```python
from build123d import *

# Parameters (mm, degrees)
M10_CLEARANCE_HOLE2_D                     = 11
M10_CLEARANCE_HOLE2_DEPTH                 = 55.695266595
M10_CLEARANCE_HOLE2_CSINK_D               = 11.05
M10_CLEARANCE_HOLE2_CSINK_ANGLE           = 90
M10_CLEARANCE_HOLE2_TIP                   = 3.304733405
M10_CLEARANCE_HOLE2_ON_FACE_2_D           = 11
M10_CLEARANCE_HOLE2_ON_FACE_2_DEPTH       = 55.695266595
M10_CLEARANCE_HOLE2_ON_FACE_2_CSINK_D     = 11.05
M10_CLEARANCE_HOLE2_ON_FACE_2_CSINK_ANGLE = 90
M10_CLEARANCE_HOLE2_ON_FACE_2_TIP         = 3.304733405
CHAMFER1_SIZE                             = 0.5


with BuildPart() as part:
    # Sketch1 → Revolve1 (revolve)
    with BuildSketch(Plane(origin=(0, 0, 0), x_dir=(0, 0, -1), z_dir=(1, 0, 0)), mode=Mode.PRIVATE) as revolve1_sk:
        Polygon((-100, 0), (100, 0), (100, 12.5), (83.5, 12.5), (79.023440019, 63.66731472), (77.097512539, 65.967489352), (-77.097512539, 65.967489352), (-79.023440019, 63.66731472), (-83.5, 12.5), (-100, 12.5), align=None)
    revolve(revolve1_sk.sketch.rotate(Axis((0, 0, 100), (0, 0, -1)), 90), axis=Axis((0, 0, 100), (0, 0, -1)))

    # M10 Clearance Hole2
    with Locations(Plane(origin=(0, 0, -100), x_dir=(-1, 0, 0), z_dir=(0, 0, -1))):
        with Locations((0, 0)):
            CounterSinkHole(M10_CLEARANCE_HOLE2_D / 2, M10_CLEARANCE_HOLE2_CSINK_D / 2, depth=M10_CLEARANCE_HOLE2_DEPTH, counter_sink_angle=M10_CLEARANCE_HOLE2_CSINK_ANGLE)
            with Locations((0, 0, -(M10_CLEARANCE_HOLE2_DEPTH + M10_CLEARANCE_HOLE2_TIP / 2))):  # 118° drill point
                Cone(0, M10_CLEARANCE_HOLE2_D / 2, M10_CLEARANCE_HOLE2_TIP, mode=Mode.SUBTRACT)

    # M10 Clearance Hole2 on face 2
    with Locations(Plane.XY.offset(100)):
        with Locations((0, 0)):
            CounterSinkHole(M10_CLEARANCE_HOLE2_ON_FACE_2_D / 2, M10_CLEARANCE_HOLE2_ON_FACE_2_CSINK_D / 2, depth=M10_CLEARANCE_HOLE2_ON_FACE_2_DEPTH, counter_sink_angle=M10_CLEARANCE_HOLE2_ON_FACE_2_CSINK_ANGLE)
            with Locations((0, 0, -(M10_CLEARANCE_HOLE2_ON_FACE_2_DEPTH + M10_CLEARANCE_HOLE2_ON_FACE_2_TIP / 2))):  # 118° drill point
                Cone(0, M10_CLEARANCE_HOLE2_ON_FACE_2_D / 2, M10_CLEARANCE_HOLE2_ON_FACE_2_TIP, mode=Mode.SUBTRACT)

    # Chamfer1
    chamfer1_edges = [part.edges().sort_by_distance(p)[0] for p in [
        (-12.5, 0, -100),
        (-12.5, 0, 100),
    ]]
    chamfer(chamfer1_edges, length=CHAMFER1_SIZE)


solid = part.part
```
Read the model definition and answer for the solid it produces. Units are mm, in the model's axes. A direction names the side the tool comes from. Give positions to 0.01 mm unless a question says otherwise; leave off trailing zeros. Order: outer loops, then holes, each group sorted by start corner. A loop starts at its lowest first (then second) coordinate and runs counter-clockwise, first axis right, second up. Notation, with made-up numbers: (67.5, -1) -> (78.5, -1) arc R25 ccw to (78.5, 36) -> close; hole circle Ø10 at (-17, 56). An arc over 180 degrees is marked (long way). Write item = value, one per line.
1. A cutting plane is placed at B-B, the plane z = -25. Write down the section's boundary in (x, y).
Numbers:
outline = circle Ø131.93 at (0, 0)
2. For faces 1 (the face through (11.923, -3.755, 91.612)), 2 (the face through (-1.19, -5.37, -71.75)), 3 (the face through (62.921, -19.815, 1.079)), determine the directions among +Z, -Z, +X, -X, +Y, -Y from which every point of the face is accessible in a straight line to the end or side of a thin tool.
Numbers:
face_1 = +Z
face_2 = -Z
face_3 = +Z, -Z
3. Straight lines are drawn through the part: line 1 along Y through (x, z) = (0, 72.5); line 2 along X through (y, z) = (-2.5, -88); line 3 along Z through (x, y) = (-19, 22). For each, find the intervals that lie inside material, in ascending order.
Numbers:
line_1 = -65.97 to -5.5, 5.5 to 65.97
line_2 = -12.25 to -4.9, 4.9 to 12.25
line_3 = -82.05 to 82.05
4. A cutting plane is placed at A-A, the plane z = -67. Write down the section's boundary in (x, y).
Numbers:
outline = circle Ø131.93 at (0, 0); hole circle Ø11 at (0, 0)
5. Given pin 1 (6.5 mm diameter, centred on x = 0, y = 0, fed in from +Z); pin 2 (1.5 mm diameter, centred on x = 10, y = 34.5, fed in from +Z); pin 3 (1.5 mm diameter, centred on x = 43.5, z = 76.5, fed in from +Y), each flat-ended and moving along its own axis, determine where each tip first touches the part or whether it passes through.
Numbers:
pin_1 = 42.95
pin_2 = 81.52
pin_3 = 50.24
6. The mould has two halves that part along X. Classify faces 4 (the face through (-5.2, 2.5, -100)), 5 (the face through (1.19, -5.37, 71.75)), 6 (the face through (60.865, -19.167, -78.903)): +X half, -X half, draft (parallel to the pull), parting line (faces both ways), or undercut.
Numbers:
face_4 = draft
face_5 = undercut
face_6 = parting line
